from build123d import *

# Parameters (mm, degrees)
F2_DEPTH = 10
F3_DEPTH = 10
F4_DEPTH = 1


with BuildPart() as f1:
    # F0 (on Front) → F1 (revolve)
    with BuildSketch(Plane.XZ):
        with BuildLine():
            Line((1.55, 2), (1.55, 0))
            Line((1.55, 0), (6.55, 0))
            Line((6.55, 0), (6.55, 14.9455200697))
            Line((6.55, 14.9455200697), (6.55, 15.9468985058))
            ThreePointArc((6.55, 15.9468985058), (19.5204691227, 13.0387576646), (30.7963834074, 6))
            Line((30.7963834074, 6), (32.2785816747, 6))
            ThreePointArc((32.2785816747, 6), (19.4618650437, 14.1407042674), (4.55, 17))
            Line((4.55, 17), (4.55, 16))
            Line((4.55, 16), (4.55, 15))
            Line((4.55, 15), (4.55, 2))
            Line((4.55, 2), (1.55, 2))
        make_face()
    revolve(axis=Axis((0, 0, 13.7464413419), (0, 0, 1)))

    # F2 (add): a face of the model
    f2_faces = [f1.faces().sort_by_distance(p)[0] for p in [
        (-1.7352619767, 0, 0),
    ]]
    extrude(f2_faces, amount=F2_DEPTH)

    # F3 (cut): a face of the model
    f3_faces = [f1.faces().sort_by_distance(p)[0] for p in [
        (-4.4213065658, 0, 2),
    ]]
    extrude(f3_faces, amount=-F3_DEPTH, mode=Mode.SUBTRACT)

    # F4 (cut): a face of the model
    f4_faces = [f1.faces().sort_by_distance(p)[0] for p in [
        (-1.7352619767, 0, -10),
    ]]
    extrude(f4_faces, amount=-F4_DEPTH, mode=Mode.SUBTRACT)


solid = f1.part
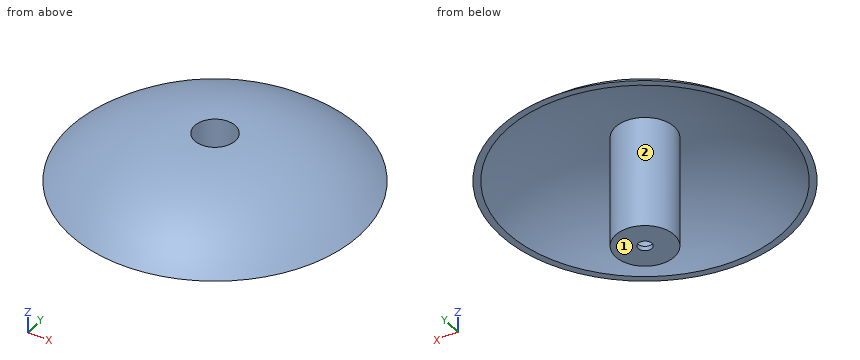
Read the model definition and answer for the solid it produces. Units are mm, in the model's axes. Face numbers are marked on the shaded views. Give positions to 0.01 mm unless a question says otherwise; leave off trailing zeros. Write each loop counter-clockwise with the first axis right and the second up, starting at its lowest first coordinate (ties: lowest second). Pieces come first, ordered by that corner, then holes. Notation, with made-up numbers: M -3,69.5 L 21,69.5 A17 cw 21,87.5 Z; hole C 30,30.5 d2. An arc over 180 degrees is marked long. One line per item, written item: value. Start each with the question number.
(1) Find section B-B (z = 8.5). Give the number of separate pieces and of enclosed holes in the cut face, plus the area to 3 significant figures.
(2) Flat-ended cylindrical pins translate along their axes: pin 1 Ø10 at (x, y) = (19, -19) entering from -Z; pin 2 Ø5 at (x, y) = (10, -19.5) entering from -Z; pin 3 Ø2.5 at (x, y) = (-1.5, 1.5) entering from +Z; pin 4 Ø10 at (y, z) = (-17.5, -1.5) entering from -X. Find the tip coordinate at first contact, or state that the pin passes through.
(3) Determine the mould class of the marked faces 1 and 2 for opening direction Y: pulls with the +Y half, pulls with the -Y half, needs draft (parallel to the pull), parting line crosses it, or undercut.
(4) Find the intervals of material crossed by line 1 (Y direction, x = 0, z = -8.4); line 2 (Y direction, x = 0, z = -5); line 3 (Y direction, x = 4, z = 8.75), in increasing order.
(5) Find section A-A (z = -7). Determine the outline of the cut face in (x, y).
Results below:
1. separate pieces: 2
1. enclosed holes: 2
1. area: 369 mm^2
2. pin 1: stops at z = 6
2. pin 2: stops at z = 10.62
2. pin 3: stops at z = -8
2. pin 4: passes through
3. face 1: needs draft
3. face 2: undercut
4. line 1: y = -6.55 to -1.55, 1.55 to 6.55
4. line 2: y = -6.55 to -4.55, 4.55 to 6.55
4. line 3: y = -28.75 to -27.04, -5.19 to -2.17, 2.17 to 5.19, 27.04 to 28.75
5. outline: C 0,0 d13.1; hole C 0,0 d9.1
